from build123d import *

# Parameters (mm, degrees)
F0_W     = 15.5
F0_H     = 31
F1_DEPTH = 5
F2_R     = 0.564605
F3_DEPTH = 4
F5_DEPTH = 2


with BuildPart() as f1:
    # F0 (on Top) → F1 (new body)
    with BuildSketch(Plane.XY):
        with Locations((7.75, -15.5)):
            Rectangle(F0_W, F0_H)
    extrude(amount=F1_DEPTH)

    # F2 (on face) → F3 (join)
    with BuildSketch(Plane(origin=(0, 0, 0), x_dir=(1, 0, 0), z_dir=(0, 0, -1))):
        with Locations((1.347199, 21.362342)):
            Circle(F2_R)
        with Locations((1.347199, 18.796942)):
            Circle(F2_R)
        with Locations((1.347199, 16.231542)):
            Circle(F2_R)
        with Locations((1.347199, 13.666142)):
            Circle(F2_R)
        with Locations((1.347199, 11.100742)):
            Circle(F2_R)
        with Locations((14.199599, 21.362342)):
            Circle(F2_R)
        with Locations((14.199599, 18.796942)):
            Circle(F2_R)
        with Locations((14.199599, 16.231542)):
            Circle(F2_R)
        with Locations((14.199599, 13.666142)):
            Circle(F2_R)
        with Locations((14.199599, 11.100742)):
            Circle(F2_R)
    extrude(amount=F3_DEPTH)

    # F4 (on face) → F5 (cut)
    with BuildSketch(Plane.XY.offset(5)):
        Polygon((4.07275, -5.926542), (4.07275, 0), (0, 0), (0, -31), (15.5, -31), (15.5, 0), (11.611941, 0), (11.611941, -5.926542), align=None)
    extrude(amount=-F5_DEPTH, mode=Mode.SUBTRACT)


solid = f1.part
Input: part model. Units: mm. Frame: model coordinates. A direction names the side the tool comes from. Coordinates: 2 decimals unless noted, no trailing zeros. Loops run counter-clockwise (first coordinate to the right, second up) from the corner with the lowest first, then second, coordinate; pieces in that order, holes last. Notation, with made-up numbers: (34, 8) -> (70, 8) arc R24 ccw to (70, 47) -> close; hole circle Ø1 at (35, 42.5). An arc over 180 degrees is marked (long way). Write item = value, one per line. Start each with the question number.
Item 1: Reachability of faces 4 (the face through (11.612, -3, 4)), 5 (the face through (0, -16, 1)), 6 (the face through (14.46, -15.73, -1.97)) from +Z, -Z, +X, -X, +Y, -Y: full face, straight path, thin tool, end or side. Return the list, or none.
Item 2: Cut plane A-A, the plane z = -1. Count the separate pieces of the cut face and the enclosed holes in it, plus the area to 3 significant figures.
Item 3: Cut plane D-D, the plane x = 2.75. Return loops of the section in (y, z).
Item 4: Cut plane B-B, the plane y = -5. Return loops of the section in (x, z).
Item 5: Material intervals for line 1 (Y direction, x = 1.75, z = -2.5); line 2 (Z direction, x = 6.75, y = -20); line 3 (Y direction, x = 14, z = -0.25), sorted ascending.
Item 6: Mould query, pull axis X, two halves, no side actions, for faces 1 (the face through (15.5, -16, 1)), 2 (the face through (14.74, -11.27, -1.97)), 3 (the face through (8, 0, 2)). Classes: pulls with the +X half, pulls with the -X half, needs draft (parallel to the pull), parting line crosses it, or undercut.
Item 7: Cut plane C-C, the plane x = 7.5. Return loops of the section in (y, z), plus the area to 3 significant figures.
Item 8: First-contact query: P1, Ø6, axis at x = 6, y = -12.5, coming from the -Z side; P2, Ø1.5, axis at x = 2, y = -8, coming from the +Z side; P3, Ø1, axis at y = -3.5, z = 4, coming from the +X side. Flat tips, straight axial feed; report the tip coordinate or a pass-through.
Ans:
q1.face_4 = +Z, +X, +Y, -Y
q1.face_5 = +Z, -Z, -X, +Y, -Y
q1.face_6 = -Z
q2.separate_pieces = 10
q2.enclosed_holes = 0
q2.area = 10.0 mm²
q3.outline = (-31, 0) -> (0, 0) -> (0, 3) -> (-31, 3) -> close
q4.outline = (0, 0) -> (15.5, 0) -> (15.5, 3) -> (11.61, 3) -> (11.61, 5) -> (4.07, 5) -> (4.07, 3) -> (0, 3) -> close
q5.line_1 = -21.76 to -20.97, -19.19 to -18.4, -16.63 to -15.84, -14.06 to -13.27, -11.5 to -10.71
q5.line_2 = 0 to 3
q5.line_3 = -21.89 to -20.83, -19.33 to -18.27, -16.76 to -15.7, -14.19 to -13.14, -11.63 to -10.57
q6.face_1 = pulls with the +X half
q6.face_2 = undercut
q6.face_3 = needs draft
q7.outline = (-31, 0) -> (0, 0) -> (0, 5) -> (-5.93, 5) -> (-5.93, 3) -> (-31, 3) -> close
q7.area = 105 mm²
q8.P1 = 0
q8.P2 = 3
q8.P3 = 11.61
